CAD build for the part. Positions are in the model's coordinates, mm. Face numbers are marked on the shaded views. Round coordinates to 2 decimals unless told otherwise and drop trailing zeros. Write each loop counter-clockwise with the first axis right and the second up, starting at its lowest first coordinate (ties: lowest second). Pieces come first, ordered by that corner, then holes. Notation, with made-up numbers: (-3.5, 21.5) -> (37.5, 21.5) arc R19 cw to (37.5, 53.5) -> close; hole circle Ø5 at (31, 15.25). An arc over 180 degrees is marked (long way). Put each result on its own line as item: value. Start each with the question number.
1. Saw through at D-D on z = -23. List the corners of the cut face in (x, y).
2. Flat gauge pins, fed straight in: P1, Ø18.5, axis at x = 14, y = -1, coming from the +Z side; P2, Ø8, axis at y = 10, z = -8.5, coming from the +X side; P3, Ø4.5, axis at x = 0, y = 0, coming from the +Z side. Where does each tip first touch, or does it go through?
3. Drill centre lines: line 1 (Y direction, x = 0, z = -14.5); line 2 (Y direction, x = 0, z = -7.25). Where is each one in solid material? Low to high. Write a range as from..to.
4. Saw through at A-A on x = 0. List the corners of the cut face in (y, z) (3 decimals), and give its area (3 significant figures).
5. Pull direction X, two halves, no side cores. Call the marked faces 1, 2 and 3: pulls with the +X half, pulls with the -X half, needs draft (parallel to the pull), parting line crosses it, or undercut.
6. Saw through at C-C on z = -12.5. List the corners of the cut face in (x, y).
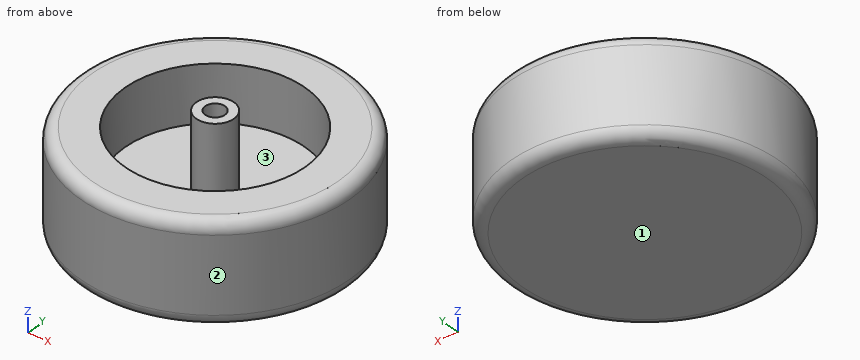
from build123d import *

# Parameters (mm, degrees)
FILLET1_R          = 3
SKETCH2_R          = 2.5
CUT_EXTRUDE1_DEPTH = 10


with BuildPart() as part:
    # Sketch1 → Revolve1 (revolve)
    with BuildSketch(Plane(origin=(0, 0, 0), x_dir=(1, 0, 0), z_dir=(0, 1, 0))):
        Polygon((0, 0), (0, 29), (34, 29), (34, 4), (22.75, 4), (22.75, 18.125), (4.75, 18.125), (4.75, 0), align=None)
    revolve(axis=Axis((0, 0, 0), (0, 0, -1)))

    # Fillet1
    fillet1_edges = [part.edges().sort_by_distance(p)[0] for p in [
        (-34, 0, -4),
        (-34, 0, -29),
    ]]
    fillet(fillet1_edges, radius=FILLET1_R)

    # Sketch2 → Cut-Extrude1 (cut)
    with BuildSketch(Plane.XY):
        Circle(SKETCH2_R)
    extrude(amount=-CUT_EXTRUDE1_DEPTH, mode=Mode.SUBTRACT)


solid = part.part
Return value:
1. outline: circle Ø68 at (0, 0)
2. P1: stops at z = -4
2. P2: stops at x = 33.47
2. P3: stops at z = -10
3. line 1: y = -34..-22.75, -4.75..4.75, 22.75..34
3. line 2: y = -34..-22.75, -4.75..-2.5, 2.5..4.75, 22.75..34
4. outline: (-34, -26) arc R3 ccw to (-31, -29) -> (31, -29) arc R3 ccw to (34, -26) -> (34, -7) arc R3 ccw to (31, -4) -> (22.75, -4) -> (22.75, -18.125) -> (4.75, -18.125) -> (4.75, 0) -> (2.5, 0) -> (2.5, -10) -> (-2.5, -10) -> (-2.5, 0) -> (-4.75, 0) -> (-4.75, -18.125) -> (-22.75, -18.125) -> (-22.75, -4) -> (-31, -4) arc R3 ccw to (-34, -7) -> close
4. area: 1,170 mm^2
5. face 1: needs draft
5. face 2: parting line crosses it
5. face 3: undercut
6. outline: circle Ø68 at (0, 0); circle Ø9.5 at (0, 0); hole circle Ø45.5 at (0, 0)
